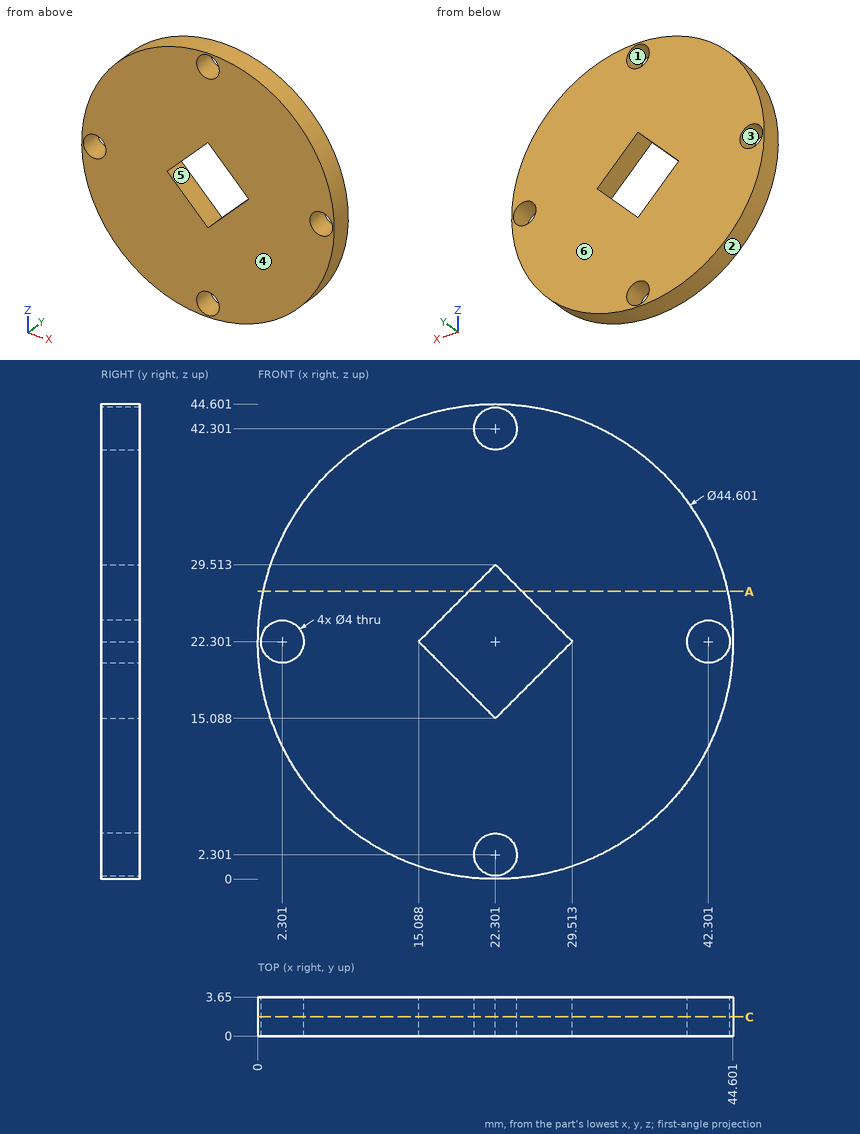
Print and shaded views of the part. All mm, measured from the part's lowest x, y and z. A direction names the side the tool comes from. Coordinates: 2 decimals unless noted, no trailing zeros. Order: outer loops, then holes, each group sorted by start corner. A loop starts at its lowest first (then second) coordinate and runs counter-clockwise, first axis right, second up.
Item 1: Saw through at C-C on y = 1.8. List the corners of the cut face in (x, z), then the cut area to 3 significant figures.
Filled in:
outline: circle Ø44.6 at (22.3, 22.3); hole circle Ø4 at (2.3, 22.3); hole (15.09, 22.3) - (22.3, 15.09) - (29.51, 22.3) - (22.3, 29.51) - close; hole circle Ø4 at (22.3, 2.3); hole circle Ø4 at (22.3, 42.3); hole circle Ø4 at (42.3, 22.3)
area: 1,410 mm2
Item 2: Drill centre lines: L1, parallel to Z at x = 23, y = 0.45 (1 decimal); L2, parallel to Z at x = 26, y = 0.35 (1 decimal); L3, parallel to X at y = 0.65, z = 19 (1 decimal). Where is each one in solid material? Low to high.
Filled in:
L1: z = 0 to 0.4, 4.2 to 15.8, 28.8 to 40.4, 44.2 to 44.6
L2: z = 0.3 to 18.8, 25.8 to 44.3
L3: x = 0.2 to 18.4, 26.2 to 44.4
Item 3: Saw through at A-A on z = 27. List the corners of the cut face in (x, y).
Filled in:
outline: (0.5, 0) - (19.79, 0) - (19.79, 3.65) - (0.5, 3.65) - close; (24.81, 0) - (44.1, 0) - (44.1, 3.65) - (24.81, 3.65) - close
Item 4: Drop flat-ended pins along their axis: pin 1 Ø2.5 at (x, z) = (2.3, 22.3) entering from +Y; pin 2 Ø5 at (x, z) = (22.3, 2.3) entering from -Y; pin 3 Ø1.5 at (y, z) = (3, 22) entering from -X. Give the stop position or say it passes through.
Filled in:
pin 1: passes through
pin 2: stops at y = 0
pin 3: stops at x = 0
Item 5: Mould opens along Z. For the marked faces 1, 2, 3 and 4 say: released by +Z, released by -Z, zero draft, split by the parting line, or undercut.
Filled in:
face 1: undercut
face 2: split by the parting line
face 3: undercut
face 4: zero draft
Item 6: Tool access for the marked faces 5 and 6: list every direction of +Z, -Z, +X, -X, +Y, -Y with a clear straight run to the whole face (end or side of a thin tool).
Filled in:
face 5: +Y, -Y
face 6: +Z, -Z, +X, -X, +Y
